Geometry: final body of the model. Coordinates: model frame, mm. Face numbers are marked on the shaded views. A direction names the side the tool comes from. Round coordinates to 2 decimals unless told otherwise and drop trailing zeros. Loops run counter-clockwise (first coordinate to the right, second up) from the corner with the lowest first, then second, coordinate; pieces in that order, holes last. Notation, with made-up numbers: M -38.5,11.5 L 14.5,11.5 A18 cw 14.5,22.5 Z; hole C 9,60.5 d9. An arc over 180 degrees is marked long. Answer as a JSON object with one key per item and string values.
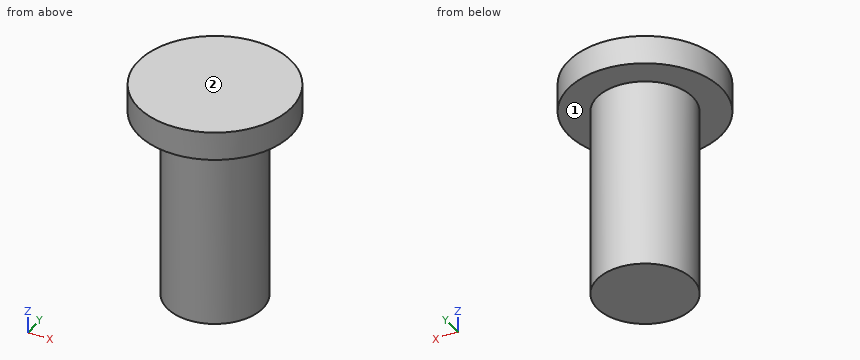
from build123d import *

# Parameters (mm, degrees)
SKETCH1_R           = 8
BOSS_EXTRUDE1_DEPTH = 3
SKETCH2_R           = 5
BOSS_EXTRUDE2_DEPTH = 10
SKETCH3_R           = 5
BOSS_EXTRUDE3_DEPTH = 10


with BuildPart() as part:
    # Sketch1 → Boss-Extrude1 (new body)
    with BuildSketch(Plane.XY):
        Circle(SKETCH1_R)
    extrude(amount=BOSS_EXTRUDE1_DEPTH)

    # Sketch2 → Boss-Extrude2 (add)
    with BuildSketch(Plane(origin=(0, 0, 0), x_dir=(-1, 0, 0), z_dir=(0, 0, -1))):
        Circle(SKETCH2_R)
    extrude(amount=BOSS_EXTRUDE2_DEPTH)

    # Sketch3 → Boss-Extrude3 (add)
    with BuildSketch(Plane(origin=(0, 0, -10), x_dir=(-1, 0, 0), z_dir=(0, 0, -1))):
        Circle(SKETCH3_R)
    extrude(amount=BOSS_EXTRUDE3_DEPTH)


solid = part.part
1) Section query D-D (y = 6). Return the cut outline in (x, z).
Results:
{"outline": "M -5.29,0 L 5.29,0 L 5.29,3 L -5.29,3 Z"}
2) Pin query (flat end, axial travel): P1, Ø5, axis at y = 3.5, z = -11, coming from the +X side; P2, Ø5, axis at y = 3.5, z = -0.5, coming from the -X side; P3, Ø5, axis at x = -1, z = -9, coming from the +Y side. Return the tip coordinate at first contact, or that it passes through.
Results:
{"P1": "x = 4.9", "P2": "x = -7.93", "P3": "y = 5"}
3) Ray query, line 1 (X direction, y = 6.25, z = 1.5); line 2 (Z direction, x = 1.5, y = -6); line 3 (Y direction, x = -1.5, z = -12.25). Return the intervals inside material, ascending.
Results:
{"line 1": "-4.99 to 4.99", "line 2": "0 to 3", "line 3": "-4.77 to 4.77"}
4) Section query A-A (x = 0). Return the cut outline in (y, z).
Results:
{"outline": "M -8,0 L -5,0 L -5,-20 L 5,-20 L 5,0 L 8,0 L 8,3 L -8,3 Z"}
5) Section query C-C (z = -9.75). Return the cut outline in (x, y).
Results:
{"outline": "C 0,0 d10"}
6) Reachability of the marked faces 1 and 2 from +Z, -Z, +X, -X, +Y, -Y: full face, straight path, thin tool, end or side. Return the list, or none.
Results:
{"face 1": "-Z", "face 2": "+Z, +X, -X, +Y, -Y"}
